Work out the finished part from the listing and answer in its coordinate system (mm). Round coordinates to 2 decimals unless told otherwise and drop trailing zeros. Order: outer loops, then holes, each group sorted by start corner. A loop starts at its lowest first (then second) coordinate and runs counter-clockwise, first axis right, second up. Notation, with made-up numbers: M 73,57 L 90,57 A16 ccw 90,85 Z; hole C 55.25,34.25 d3. An arc over 180 degrees is marked long. Answer as a JSON object with one key per item and string values. Group by question number.
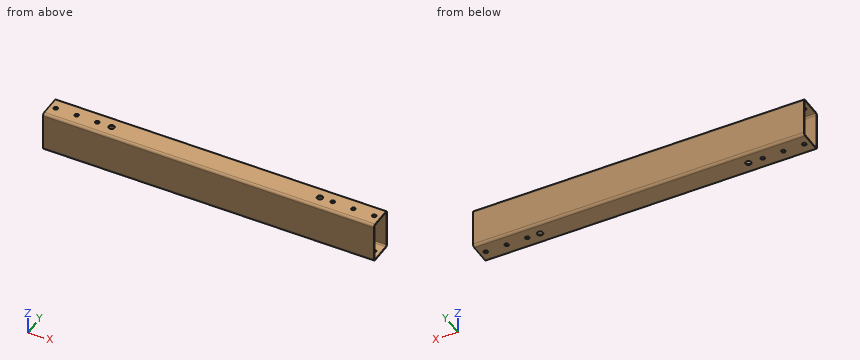
from build123d import *

# Parameters (mm, degrees)
TUBO_RETANGULAR_50_X_30_X_2_6_1_DEPTH = 405.6
ESBO_O2_R                             = 2.5
CORTE_EXTRUS_O1_DEPTH                 = 409.945424232
ESBO_O3_R                             = 3.5
CORTE_EXTRUS_O2_DEPTH                 = 409.945424232


with BuildPart() as part:
    # Sketch1 → Tubo retangular 50 X 30 X 2.6(1) (new body)
    with BuildSketch(Plane.YZ):
        with BuildLine():
            Line((-12, -25), (12, -25))
            ThreePointArc((12, -25), (14.121320344, -24.121320344), (15, -22))
            Line((15, -22), (15, 22))
            ThreePointArc((15, 22), (14.121320344, 24.121320344), (12, 25))
            Line((12, 25), (-12, 25))
            ThreePointArc((-12, 25), (-14.121320344, 24.121320344), (-15, 22))
            Line((-15, 22), (-15, -22))
            ThreePointArc((-15, -22), (-14.121320344, -24.121320344), (-12, -25))
        make_face()
        with BuildLine():
            Line((-12, -23.8), (12, -23.8))
            ThreePointArc((12, -23.8), (13.272792206, -23.272792206), (13.8, -22))
            Line((13.8, -22), (13.8, 22))
            ThreePointArc((13.8, 22), (13.272792206, 23.272792206), (12, 23.8))
            Line((12, 23.8), (-12, 23.8))
            ThreePointArc((-12, 23.8), (-13.272792206, 23.272792206), (-13.8, 22))
            Line((-13.8, 22), (-13.8, -22))
            ThreePointArc((-13.8, -22), (-13.272792206, -23.272792206), (-12, -23.8))
        make_face(mode=Mode.SUBTRACT)
    extrude(amount=TUBO_RETANGULAR_50_X_30_X_2_6_1_DEPTH)

    # Esboço2 → Corte-extrusão1 (cut, through all)
    with BuildSketch(Plane(origin=(0, 0, -25), x_dir=(-1, 0, 0), z_dir=(0, 0, -1))):
        with Locations((-58.5, 0)):
            Circle(ESBO_O2_R)
        with Locations((-33.1, 0)):
            Circle(ESBO_O2_R)
        with Locations((-7.7, 0)):
            Circle(ESBO_O2_R)
        with Locations(Location((-397.9, 0, 0), (0, 0, 180))):
            Circle(ESBO_O2_R)
        with Locations(Location((-372.5, 0, 0), (0, 0, 180))):
            Circle(ESBO_O2_R)
        with Locations(Location((-347.1, 0, 0), (0, 0, 180))):
            Circle(ESBO_O2_R)
    extrude(amount=-CORTE_EXTRUS_O1_DEPTH, mode=Mode.SUBTRACT)

    # Esboço3 → Corte-extrusão2 (cut, through all)
    with BuildSketch(Plane.XY.offset(25)):
        with Locations((75.984705047, 0)):
            Circle(ESBO_O3_R)
        with Locations((331.384705047, 0)):
            Circle(ESBO_O3_R)
    extrude(amount=-CORTE_EXTRUS_O2_DEPTH, mode=Mode.SUBTRACT)


solid = part.part
Item 1: Find section B-B (x = 242). Give the vertices of the cut face in (y, z).
Item 2: Consider L1, parallel to Y at x = 274, z = 6.5; L2, parallel to Z at x = 101, y = -5; L3, parallel to Y at x = 347, z = -24. Determine where each line is inside the solid, lowest interval first.
Item 3: Find section C-C (y = -8.5). Give the vertices of the cut face in (x, z), and give its area (3 significant figures).
Item 4: Find section A-A (z = -12). Give the vertices of the cut face in (x, y).
Responses:
{
 "1": {"outline": "M -15,-22 A3 ccw -12,-25 L 12,-25 A3 ccw 15,-22 L 15,22 A3 ccw 12,25 L -12,25 A3 ccw -15,22 Z; hole M -13.8,-22 A1.8 ccw -12,-23.8 L 12,-23.8 A1.8 ccw 13.8,-22 L 13.8,22 A1.8 ccw 12,23.8 L -12,23.8 A1.8 ccw -13.8,22 Z"},
 "2": {"L1": "y = -15 to -13.8, 13.8 to 15", "L2": "z = -25 to -23.8, 23.8 to 25", "L3": "y = -14.24 to -2.5, 2.5 to 14.24"},
 "3": {"outline": "M 0,-25 L 405.6,-25 L 405.6,-23.8 L 0,-23.8 Z; M 0,23.8 L 405.6,23.8 L 405.6,25 L 0,25 Z", "area": "973 mm^2"},
 "4": {"outline": "M 0,-15 L 405.6,-15 L 405.6,-13.8 L 0,-13.8 Z; M 0,13.8 L 405.6,13.8 L 405.6,15 L 0,15 Z"}
}
